```python
from build123d import *

# Parameters (mm, degrees)
F0_R      = 7.5
F1_DEPTH  = 75
F1_FACE_R = 7.5
F4_R      = 2.5
F5_DEPTH  = 7.5
F7_D      = 5
F8_SIZE2  = 3
F8_SIZE   = 15
F9_R      = 5


with BuildPart() as f1:
    # F0 (on Front) → F1 (new body)
    with BuildSketch(Plane.XZ):
        Circle(F0_R)
    extrude(amount=F1_DEPTH)

    # F3: sweep along a path in F2
    with BuildLine(Plane.XY) as f3_path:
        Line((0, 0), (0, 100))
        Line((0, 100), (-40, 100))
    # F1_face (on face) → F3 (sweep)
    with BuildSketch(Plane(origin=(0, 0, 0), x_dir=(1, 0, 0), z_dir=(0, 1, 0))):
        Circle(F1_FACE_R)
    sweep(path=f3_path.line, transition=Transition.RIGHT)

    # F4 (on Right) → F5 (join, symmetric)
    with BuildSketch(Plane.YZ):
        Circle(F4_R)
    extrude(amount=F5_DEPTH, both=True)

    # F7 (through all)
    with Locations(Plane(origin=(-7.5, 0, 0), x_dir=(0, -1, 0), z_dir=(-1, 0, 0))):
        with Locations((0, 0)):
            Hole(F7_D / 2)

    # F8
    f8_edges = [f1.edges().sort_by_distance(p)[0] for p in [
        (-7.5, -75, 0),
    ]]
    f8_side = f1.faces().sort_by_distance((-7.5, 16.25, 0))[0]
    chamfer(f8_edges, length=F8_SIZE, length2=F8_SIZE2, reference=f8_side)

    # F9
    f9_edges = [f1.edges().sort_by_distance(p)[0] for p in [
        (-40, 92.5, 0),
    ]]
    fillet(f9_edges, radius=F9_R)


solid = f1.part
```
The listing builds one solid part. Answer for the finished solid, in the listing's coordinates (mm). Give positions to 0.01 mm unless a question says otherwise; leave off trailing zeros. Loops run counter-clockwise (first coordinate to the right, second up) from the corner with the lowest first, then second, coordinate; pieces in that order, holes last. Notation, with made-up numbers: M 10,51 L 42,51 A27 ccw 42,78 Z; hole C 32.5,43 d6. An arc over 180 degrees is marked long. One line per item, written item: value.
Q1. A cutting plane is placed at D-D on y = 0. Determine the outline of the cut face in (x, z), then the cut area to 3 significant figures.
Working result:
outline: M -7.07,-2.5 A7.5 ccw 7.07,-2.5 Z; M -7.07,2.5 L 7.07,2.5 A7.5 ccw Z
area: 103 mm^2
Q2. Flat-ended cylindrical pins translate along their axes: P1, Ø3, axis at x = -1.5, z = -4, coming from the +Y side; P2, Ø6, axis at y = -8.5, z = -3.5, coming from the -X side; P3, Ø1.5, axis at x = -27, z = -1, coming from the +Y side. Find the tip coordinate at first contact, or state that the pin passes through.
Working result:
P1: stops at y = 107.07
P2: stops at x = -7.48
P3: stops at y = 107.5
Q3. A cutting plane is placed at C-C on x = -23. Determine the outline of the cut face in (y, z).
Working result:
outline: C 100,0 d15
Q4. A cutting plane is placed at A-A on x = 0. Determine the outline of the cut face in (y, z), then the cut area to 3 significant figures.
Working result:
outline: M -75,-4.5 L -60,-7.5 L 100,-7.5 A7.5 ccw 100,7.5 L -60,7.5 L -75,4.5 Z; hole C 0,0 d5
area: 2,650 mm^2
Q5. A cutting plane is placed at B-B on y = -42.5. Determine the outline of the cut face in (x, z).
Working result:
outline: C 0,0 d15
Q6. Find the intervals of material crossed by line 1 (Z direction, x = 2, y = 0.5); line 2 (X direction, y = -39.5, z = 6); line 3 (Z direction, x = -4, y = 0), in increasing order. Write a range as from..to.
Working result:
line 1: z = -7.23..-2.45, 2.45..7.23
line 2: x = -4.5..4.5
line 3: z = -6.34..-2.5, 2.5..6.34
Q7. Determine the mould class of faces 1 (the face through (-18.77, 107.154, -2.253)), 2 (the face through (5.385, -69.272, 1.696)), 3 (the face through (0.1, -0.54, -2.44)), 4 (the face through (7.154, 24.922, -2.253)) for opening direction Y: +Y half, -Y half, draft (parallel to the pull), parting line (faces both ways), or undercut.
Working result:
face 1: parting line
face 2: -Y half
face 3: undercut
face 4: draft
